from build123d import *

# Parameters (mm, degrees)
SKETCH_1_R          = 49
EXTRUDE_1_DEPTH     = 8
SKETCH_2_R          = 31
EXTRUDE_2_DEPTH     = 10
SKETCH_3_R          = 25
CUT_EXTRUDE_1_DEPTH = 9
SKETCH_4_R          = 4.5
CUT_EXTRUDE_2_DEPTH = 49


with BuildPart() as part:
    # 草图1 → 凸台-拉伸1 (new body)
    with BuildSketch(Plane.XY):
        Circle(SKETCH_1_R)
    extrude(amount=EXTRUDE_1_DEPTH)

    # 草图2 → 凸台-拉伸2 (add)
    with BuildSketch(Plane.XY.offset(8)):
        Circle(SKETCH_2_R)
    extrude(amount=EXTRUDE_2_DEPTH)

    # 草图3 → 切除-拉伸1 (cut)
    with BuildSketch(Plane.XY.offset(18)):
        Circle(SKETCH_3_R)
    extrude(amount=-CUT_EXTRUDE_1_DEPTH, mode=Mode.SUBTRACT)

    # 草图4 → 切除-拉伸2 (cut)
    with BuildSketch(Plane.XY.offset(8)):
        with Locations((0, 40)):
            Circle(SKETCH_4_R)
        with Locations((40, 0)):
            Circle(SKETCH_4_R)
        with Locations((0, -40)):
            Circle(SKETCH_4_R)
        with Locations((-40, 0)):
            Circle(SKETCH_4_R)
    extrude(amount=-CUT_EXTRUDE_2_DEPTH, mode=Mode.SUBTRACT)


solid = part.part
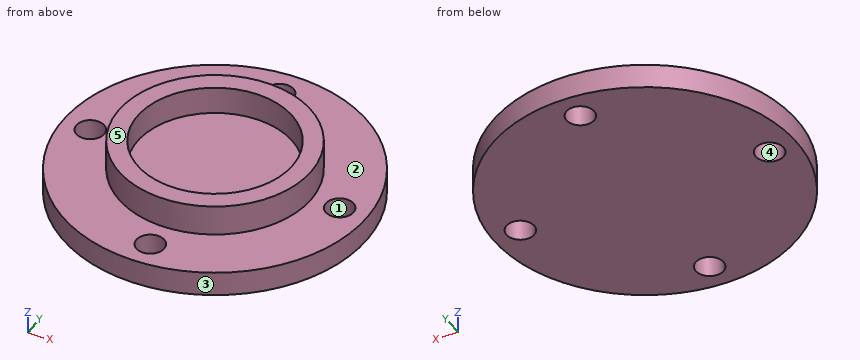
Source: CAD feature listing. Evaluate the final solid. Frame: model axes, mm. Face numbers are marked on the shaded views. A direction names the side the tool comes from. Round coordinates to 2 decimals unless told otherwise and drop trailing zeros. Loops run counter-clockwise (first coordinate to the right, second up) from the corner with the lowest first, then second, coordinate; pieces in that order, holes last. Notation, with made-up numbers: (-2, -16.75) - (56, -16.75) arc R16 cw to (56, -1.75) - close; hole circle Ø3 at (-39.5, 89). An arc over 180 degrees is marked (long way). Write item = value, one per line. Start each with the question number.
(1) Pull-direction query (X, two-part tool) for the marked faces 3, 4 and 5; classes: +X half, -X half, draft (parallel to the pull), parting line (faces both ways), or undercut.
(2) Section query B-B, the plane y = -40. Output: boundary loops of the cut face in (x, z), plus the area to 3 significant figures.
(3) Set-up query: the marked faces 1 and 2. Return all of +Z, -Z, +X, -X, +Y, -Y with unobstructed straight access to the full face (end or side cutting, diameter ignored); none if empty.
(4) Pin query (flat end, axial travel): pin 1 (8 mm diameter, centred on y = 8.5, z = 5, fed in from +X); pin 2 (8 mm diameter, centred on x = -9.5, y = -17.5, fed in from +Z); pin 3 (5.5 mm diameter, centred on x = 40, y = 0, fed in from +Z); pin 4 (1.5 mm diameter, centred on x = -13, z = 14.5, fed in from -Y). Return the tip coordinate at first contact, or that it passes through.
(5) Section query A-A, the plane x = 0. Output: boundary loops of the cut face in (y, z), plus the area to 3 significant figures.
(6) Ray query, line 1 along Y through (x, z) = (0, 13.5); line 2 along X through (y, z) = (-1.5, 6.25); line 3 along Z through (x, y) = (0, -22). Return the intervals inside material, ascending. Write a range as from..to.
(7) Section query D-D, the plane z = 12.75. Output: boundary loops of the cut face in (x, y).
Conclusion:
q1.face_3 = parting line
q1.face_4 = undercut
q1.face_5 = draft
q2.outline = (-28.3, 0) - (-4.5, 0) - (-4.5, 8) - (-28.3, 8) - close; (4.5, 0) - (28.3, 0) - (28.3, 8) - (4.5, 8) - close
q2.area = 381 mm2
q3.face_1 = +Z, -Z
q3.face_2 = +Z
q4.pin_1 = 48.79
q4.pin_2 = 9
q4.pin_3 = through
q4.pin_4 = -28.48
q5.outline = (-49, 0) - (-44.5, 0) - (-44.5, 8) - (-49, 8) - close; (-35.5, 0) - (35.5, 0) - (35.5, 8) - (31, 8) - (31, 18) - (25, 18) - (25, 9) - (-25, 9) - (-25, 18) - (-31, 18) - (-31, 8) - (-35.5, 8) - close; (44.5, 0) - (49, 0) - (49, 8) - (44.5, 8) - close
q5.area = 810 mm2
q6.line_1 = -31..-25, 25..31
q6.line_2 = -48.98..-44.24, -35.76..35.76, 44.24..48.98
q6.line_3 = 0..9
q7.outline = circle Ø62 at (0, 0); hole circle Ø50 at (0, 0)
